Check sheet for the modelled part. Datum: model origin and axes. Units: mm. Give positions to 0.01 mm unless a question says otherwise; leave off trailing zeros. Loops run counter-clockwise (first coordinate to the right, second up) from the corner with the lowest first, then second, coordinate; pieces in that order, holes last. Notation, with made-up numbers: (48, -36.5) -> (73, -36.5) arc R19 cw to (73, -2.5) -> close; hole circle Ø9 at (21, 43.25). An arc over 180 degrees is marked (long way). Write each question's results on one line, items separated by ' | '. Start each with the question number.
Item 1: Cross-section at D-D on y = 58. Enter the section's corners in (x, z) (3 decimals), then the cut area to 3 significant figures.
Item 2: Scan lines: line 1 along Y through (x, z) = (15, 2.7); line 2 along Y through (x, z) = (12.7, 2.2); line 3 along Y through (x, z) = (53.5, 0.55). Record each from-to range of solid material in increasing order.
Item 3: Gauge pin test, flat ends, axial feed: pin 1 Ø6.5 at (x, y) = (7.874, 12.7) entering from +Z; pin 2 Ø1 at (x, z) = (35, 1) entering from -Y; pin 3 Ø1 at (y, z) = (115.5, 3) entering from +X. Record the tip position at first contact, or that the pin passes through.
Item 4: Cross-section at C-C on z = 1.45. Enter the section's corners in (x, y) (3 decimals).
Item 5: Cross-section at B-B on x = 56. Enter the section's corners in (y, z) (3 decimals), then the cut area to 3 significant figures.
Item 6: Mould release check, pull along X, two halves, no side actions. Record for faces 1 (the face through (38.08, 90.09, 1.57)), 2 (the face through (9.786, 15.698, 1.61)), 3 (the face through (27, 38, 0)): pulls with the +X half, pulls with the -X half, needs draft (parallel to the pull), parting line crosses it, or undercut.
Item 7: Cross-section at A-A on y = 12.7. Enter the section's corners in (x, z) (3 decimals).
Autodesk Inventor part; units mm, degrees
ref_plane "YZ Plane" through (0, 0, 0) normal (1, 0, 0) x (0, 1, 0)
ref_plane "XZ Plane" through (0, 0, 0) normal (0, 1, 0) x (-1, 0, 0)
ref_plane "XY Plane" through (0, 0, 0) normal (0, 0, 1) x (1, 0, 0)
sketch "Sketch1" plane through (0, 0, 0) normal (0, 0, 1) x (1, 0, 0)
  line L0 (69.85, 0) -> (69.85, 38.1)
  line L1 (69.85, 38.1) -> (0, 152.4)
  line L2 (0, 152.4) -> (0, 0)
  line L3 (69.85, 0) -> (0, -76.2)
  line L4 (0, -76.2) -> (0, 0)
  dimension "d1" = 38.1
  dimension "d2" = 152.4
  dimension "d24" = 76.2
  dimension "d25" = 69.85
  dimension "d26" = 69.85
extrude "Extrusion1" add sketch "Sketch1" along normal blind 3.175
sketch "Sketch2" plane through (0, 0, 3.175) normal (0, 0, 1) x (1, 0, 0)
  line L0 (0, 0) -> (69.85, 0)
  line L1 (69.85, 0) -> (69.85, 38.1)
  line L2 (0, 152.4) -> (0, -76.2)
  circle A0 centre (7.874, 12.7) radius 3.556
  circle A1 centre (55.626, 12.7) radius 3.556
  dimension "d5" = 7.112
  dimension "d6" = 7.112
  dimension "d7" = 12.7
  dimension "d8" = 12.7
  dimension "d9" = 14.224
  dimension "d11" = 7.874
extrude "Extrusion2" cut sketch "Sketch2" against normal blind 25.4
fillet "Fillet1" radius 3.175 1 edges at (0, 152.4, 1.5875)
sketch "Sketch3" plane through (0, 0, 3.175) normal (0, 0, 1) x (1, 0, 0)
  line L0 (0, 141.1158) -> (0, -76.2)
  line L1 (0, 0) -> (69.85, 0)
  circle A0 centre (12.7, 94.9198) radius 3.3782
  circle A1 centre (12.7, 44.1198) radius 3.3782
  dimension "d15" = 6.7564
  dimension "d16" = 6.7564
  dimension "d17" = 12.7
  dimension "d18" = 12.7
  dimension "d19" = 44.1198
  dimension "d20" = 50.8
extrude "Extrusion3" cut sketch "Sketch3" against normal blind 25.4
fillet "Fillet2" radius 3.175 2 edges at (69.85, 0, 1.5875) (69.85, 38.1, 1.5875)
fillet "Fillet3" radius 3.175 1 edges at (0, -76.2, 1.5875)
sketch "Sketch4" plane through (0, 0, 3.175) normal (0, 0, 1) x (1, 0, 0)
  line L0 (0, 141.1158) -> (0, -68.0377)
  circle A0 centre (12.7, 44.1198) radius 3.3782
  circle A1 centre (12.7, -35.2552) radius 3.3782
  point P0 (0, 0)
  dimension "d28" = 6.7564
  dimension "d29" = 79.375
  dimension "d30" = 12.7
extrude "Extrusion4" cut sketch "Sketch4" against normal blind 25.4 contours A1
sketch "Sketch5" plane through (0, 0, 3.175) normal (0, 0, 1) x (1, 0, 0)
  circle A0 centre (12.7, 44.1198) radius 3.3782
  circle A1 centre (12.7, 94.9198) radius 3.3782
  point P0 (0, 0)
extrude "Extrusion5" cut sketch "Sketch5" against normal blind 25.4
properties part number "Ninja cylinder support bracket"
Answer sheet:
1) outline: (0, 0) -> (57.689, 0) -> (57.689, 3.175) -> (0, 3.175) -> close | area: 183 mm²
2) line 1: y = -59.84 to -37.73, -32.78 to 41.65, 46.59 to 92.45, 97.39 to 127.85 | line 2: y = -62.35 to -38.63, -31.88 to 40.74, 47.5 to 91.54, 98.3 to 131.62 | line 3: y = -17.84 to 9.85, 15.55 to 64.85
3) pin 1: passes through | pin 2: stops at y = -38.56 | pin 3: stops at x = 22.86
4) outline: (0, -68.038) arc R3.175 ccw to (5.515, -70.183) -> (69.015, -0.91) arc R3.175 ccw to (69.85, 1.235) -> (69.85, 37.207) arc R3.175 ccw to (69.384, 38.862) -> (5.884, 142.771) arc R3.175 ccw to (0, 141.116) -> close; hole circle Ø7.112 at (7.874, 12.7); hole circle Ø6.756 at (12.7, -35.255); hole circle Ø6.756 at (12.7, 44.12); hole circle Ø6.756 at (12.7, 94.92); hole circle Ø7.112 at (55.626, 12.7)
5) outline: (-15.109, 0) -> (9.164, 0) -> (9.164, 3.175) -> (-15.109, 3.175) -> close; (16.236, 0) -> (60.764, 0) -> (60.764, 3.175) -> (16.236, 3.175) -> close | area: 218 mm²
6) face 1: pulls with the +X half | face 2: undercut | face 3: needs draft
7) outline: (0, 0) -> (4.318, 0) -> (4.318, 3.175) -> (0, 3.175) -> close; (11.43, 0) -> (52.07, 0) -> (52.07, 3.175) -> (11.43, 3.175) -> close; (59.182, 0) -> (69.85, 0) -> (69.85, 3.175) -> (59.182, 3.175) -> close
